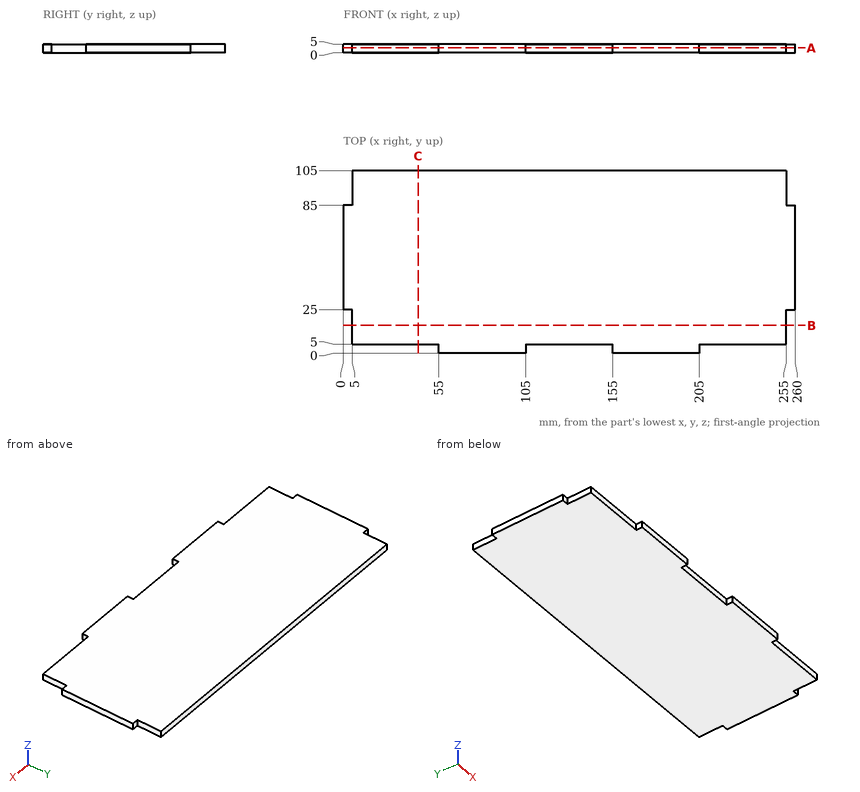
For this review, use the dimensioned drawing (mm, ordinates from the lowest corner) and the shaded views. Round coordinates to 2 decimals unless told otherwise and drop trailing zeros. Loops run counter-clockwise (first coordinate to the right, second up) from the corner with the lowest first, then second, coordinate; pieces in that order, holes last. Notation, with made-up numbers: M 12.25,-37.75 L 64.25,-37.75 A12 ccw 64.25,-29.75 Z; hole C 23.25,39 d5. An arc over 180 degrees is marked long. Answer as a JSON object with one key per item and string values.
(1) Clearance check with flat-ended pins moving along their axes: P1, Ø1.5, axis at x = 125, z = 3.5, coming from the -Y side; P2, Ø2.5, axis at x = 258, z = 2.5, coming from the +Y side; P3, Ø2.5, axis at y = 12, z = 3, coming from the -X side. State where each tip first meets the part, or that it passes through.
Resolved:
{"P1": "y = 5", "P2": "y = 85", "P3": "x = 5"}
(2) Take a section at A-A on z = 2.8. Give the boundary of the cut face in (x, y).
Resolved:
{"outline": "M 0,25 L 5,25 L 5,5 L 55,5 L 55,0 L 105,0 L 105,5 L 155,5 L 155,0 L 205,0 L 205,5 L 255,5 L 255,25 L 260,25 L 260,85 L 255,85 L 255,105 L 5,105 L 5,85 L 0,85 Z"}
(3) Take a section at B-B on y = 16. Give the boundary of the cut face in (x, z), and give its area (3 significant figures).
Resolved:
{"outline": "M 5,0 L 255,0 L 255,5 L 5,5 Z", "area": "1,250 mm²"}
(4) Take a section at C-C on x = 43. Give the boundary of the cut face in (y, z).
Resolved:
{"outline": "M 5,0 L 105,0 L 105,5 L 5,5 Z"}
(5) To check wall thickness, follow line 1 along X through (y, z) = (95.5, 0.6); line 2 along Y through (x, z) = (131, 3.6). State the ranges of each line that lie inside material, in increasing order.
Resolved:
{"line 1": "5 to 255", "line 2": "5 to 105"}
